Job drawing, mm, ordinate dimensions from the low corner. One solid piece. Round coordinates to 2 decimals unless told otherwise and drop trailing zeros. Write each loop counter-clockwise with the first axis right and the second up, starting at its lowest first coordinate (ties: lowest second). Pieces come first, ordered by that corner, then holes. Notation, with made-up numbers: M 12,18.5 L 67,18.5 A27 ccw 67,36.5 Z; hole C -34,5.25 d5. An arc over 180 degrees is marked long. Answer as a JSON object with one key per item and string values. Group by question number.
1. Band-saw the part on D-D, the plane y = 1.25. Write the cut outline in (x, z) (1 decimal).
2. Drill centre lines: line 1 (X direction, y = 8.5, z = 25.4); line 2 (Z direction, x = 22, y = 2.75); line 3 (Z direction, x = 32.5, y = 9.5). Where is each one in solid material? Low to high. Write a range as from..to.
3. Two-plate mould, pull along X, no slides. Class the marked faces 1, 2 and 3: +X half, -X half, draft (parallel to the pull), parting line (faces both ways), or undercut.
4. Band-saw the part on A-A, the plane x = 25.4. Write the cut outline in (y, z).
5. Drop a flat-ended pin along its axis: pin 1 (1.5 mm diameter, centred on x = 41, z = 24, fed in from -Y). Give the stop position or say it passes through.
6. Band-saw the part on C-C, the plane y = 10. Write the cut outline in (x, z) (1 decimal), plus the area to 3 significant figures.
7. Band-saw the part on B-B, the plane z = 25.4. Write the cut outline in (x, y).
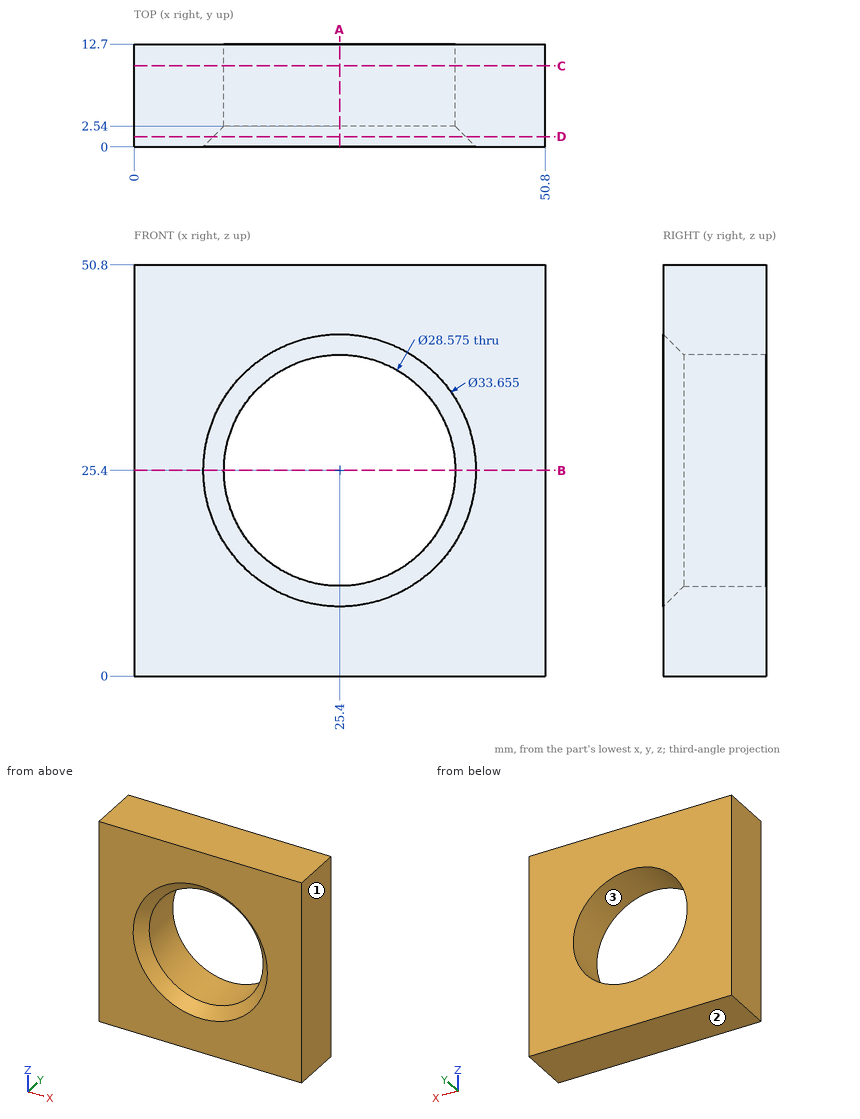
Worked answers:
{
 "1": {"outline": "M 0,0 L 50.8,0 L 50.8,50.8 L 0,50.8 Z; hole C 25.4,25.4 d31.2"},
 "2": {"line 1": "x = 0..11.11, 39.69..50.8", "line 2": "z = 0..11.52, 39.28..50.8", "line 3": "z = 0..13, 37.8..50.8"},
 "3": {"face 1": "+X half", "face 2": "draft", "face 3": "undercut"},
 "4": {"outline": "M 0,0 L 12.7,0 L 12.7,11.11 L 2.54,11.11 L 0,8.57 Z; M 0,42.23 L 2.54,39.69 L 12.7,39.69 L 12.7,50.8 L 0,50.8 Z"},
 "5": {"pin 1": "stops at y = 0.41"},
 "6": {"outline": "M 0,0 L 50.8,0 L 50.8,50.8 L 0,50.8 Z; hole C 25.4,25.4 d28.6", "area": "1,940 mm^2"},
 "7": {"outline": "M 0,0 L 8.57,0 L 11.11,2.54 L 11.11,12.7 L 0,12.7 Z; M 39.69,2.54 L 42.23,0 L 50.8,0 L 50.8,12.7 L 39.69,12.7 Z"}
}
